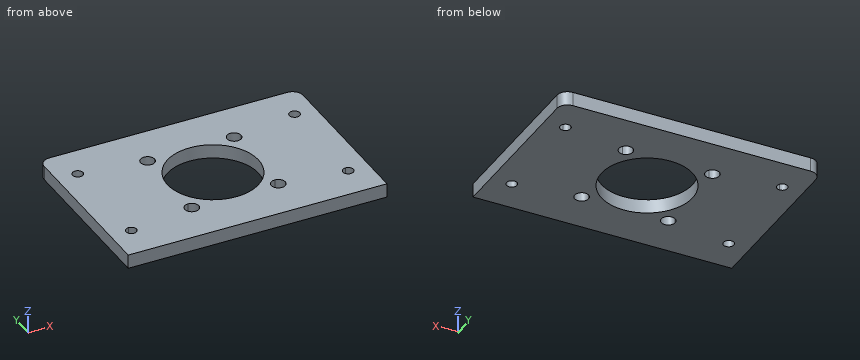
```python
from build123d import *

# Parameters (mm, degrees)
SKETCH_1_W            = 74
SKETCH_1_H            = 50
EXTRUDE_1_DEPTH       = 4
SKETCH_2_R            = 13
CUT_EXTRUDE_1_DEPTH   = 45.833023543
CUT_EXTRUDE_2_DEPTH   = 45.833023543
MIRROR_2_COPY_1_DEPTH = 45.833023543
CUT_EXTRUDE_3_DEPTH   = 45.833023543
MIRROR_4_COPY_1_DEPTH = 45.833023543
FILLET_2_R            = 3


with BuildPart() as part:
    # 草图1 → 凸台-拉伸1 (new body)
    with BuildSketch(Plane.XY):
        Rectangle(SKETCH_1_W, SKETCH_1_H)
    extrude(amount=EXTRUDE_1_DEPTH)

    # 草图2 → 切除-拉伸1 (cut, through all)
    with BuildSketch(Plane.XY.offset(4)):
        Circle(SKETCH_2_R)
    extrude(amount=-CUT_EXTRUDE_1_DEPTH, mode=Mode.SUBTRACT)

    # 草图3 → 切除-拉伸2 (cut, through all)
    with BuildSketch(Plane.XY.offset(4)):
        with BuildLine():
            ThreePointArc((10.374368671, 12.374368671), (10.960155108, 10.960155108), (12.374368671, 10.374368671))
            Line((12.374368671, 10.374368671), (12.374368671, 12.374368671))
            Line((12.374368671, 12.374368671), (10.374368671, 12.374368671))
        make_face()
        with BuildLine():
            Line((12.374368671, 12.374368671), (12.374368671, 10.374368671))
            ThreePointArc((12.374368671, 10.374368671), (13.788582233, 10.960155108), (14.374368671, 12.374368671))
            ThreePointArc((14.374368671, 12.374368671), (12.374368671, 14.374368671), (10.374368671, 12.374368671))
            Line((10.374368671, 12.374368671), (12.374368671, 12.374368671))
        make_face()
    cut_extrude_2 = extrude(amount=-CUT_EXTRUDE_2_DEPTH, mode=Mode.SUBTRACT)

    # 镜向1: 切除-拉伸2 across plane
    add(cut_extrude_2.mirror(Plane(origin=(0, 0, 0), x_dir=(0, 0, 1), z_dir=(1, 0, 0))), mode=Mode.SUBTRACT)

    # 镜向2: 切除-拉伸2 across plane
    add(cut_extrude_2.mirror(Plane.ZX), mode=Mode.SUBTRACT)

    # 镜向2 copy 1 sketch → 镜向2 copy 1 (cut, through all)
    with BuildSketch(Plane(origin=(0, 0, 4), x_dir=(-1, 0, 0), z_dir=(0, 0, 1))):
        with BuildLine():
            ThreePointArc((10.374368671, 12.374368671), (10.960155108, 10.960155108), (12.374368671, 10.374368671))
            Line((12.374368671, 10.374368671), (12.374368671, 12.374368671))
            Line((12.374368671, 12.374368671), (10.374368671, 12.374368671))
        make_face()
        with BuildLine():
            Line((12.374368671, 12.374368671), (12.374368671, 10.374368671))
            ThreePointArc((12.374368671, 10.374368671), (13.788582233, 10.960155108), (14.374368671, 12.374368671))
            ThreePointArc((14.374368671, 12.374368671), (12.374368671, 14.374368671), (10.374368671, 12.374368671))
            Line((10.374368671, 12.374368671), (12.374368671, 12.374368671))
        make_face()
    extrude(amount=-MIRROR_2_COPY_1_DEPTH, mode=Mode.SUBTRACT)

    # 草图4 → 切除-拉伸3 (cut, through all)
    with BuildSketch(Plane.XY.offset(4)):
        with BuildLine():
            ThreePointArc((-29.5, 15), (-32.060660172, 16.060660172), (-31, 13.5))
            Line((-31, 13.5), (-31, 15))
            Line((-31, 15), (-29.5, 15))
        make_face()
        with BuildLine():
            Line((-31, 15), (-31, 13.5))
            ThreePointArc((-31, 13.5), (-29.939339828, 13.939339828), (-29.5, 15))
            Line((-29.5, 15), (-31, 15))
        make_face()
    cut_extrude_3 = extrude(amount=-CUT_EXTRUDE_3_DEPTH, mode=Mode.SUBTRACT)

    # 镜向3: 切除-拉伸3 across plane
    add(cut_extrude_3.mirror(Plane(origin=(0, 0, 0), x_dir=(0, 0, 1), z_dir=(1, 0, 0))), mode=Mode.SUBTRACT)

    # 镜向4: 切除-拉伸3 across plane
    add(cut_extrude_3.mirror(Plane.ZX), mode=Mode.SUBTRACT)

    # 镜向4 copy 1 sketch → 镜向4 copy 1 (cut, through all)
    with BuildSketch(Plane(origin=(0, 0, 4), x_dir=(-1, 0, 0), z_dir=(0, 0, 1))):
        with BuildLine():
            ThreePointArc((-29.5, 15), (-32.060660172, 16.060660172), (-31, 13.5))
            Line((-31, 13.5), (-31, 15))
            Line((-31, 15), (-29.5, 15))
        make_face()
        with BuildLine():
            Line((-31, 15), (-31, 13.5))
            ThreePointArc((-31, 13.5), (-29.939339828, 13.939339828), (-29.5, 15))
            Line((-29.5, 15), (-31, 15))
        make_face()
    extrude(amount=-MIRROR_4_COPY_1_DEPTH, mode=Mode.SUBTRACT)

    # 圆角2
    fillet_2_edges = [part.edges().sort_by_distance(p)[0] for p in [
        (-37, 25, 2),
        (37, 25, 2),
    ]]
    fillet(fillet_2_edges, radius=FILLET_2_R)


solid = part.part
```
For this review, take the finished solid that the model builds, in its own axes (mm). Round coordinates to 2 decimals unless told otherwise and drop trailing zeros. Write each loop counter-clockwise with the first axis right and the second up, starting at its lowest first coordinate (ties: lowest second). Pieces come first, ordered by that corner, then holes. Notation, with made-up numbers: (-14.75, -39) -> (20.25, -39) arc R10 ccw to (20.25, -26) -> close; hole circle Ø8 at (-15.5, 35). An arc over 180 degrees is marked (long way). One line per question, with ' | ' between items. Start each with the question number.
(1) Add section A-A, the plane z = 0.75. Give the number of separate pieces and of enclosed holes in the cut face, plus the area to 3 significant figures.
(2) Insertion check: P1, Ø6, axis at x = 3, y = 11.5, coming from the -Z side. The pin has a flat end and moves straight along its axis. Give the tip position at first contact, or say it passes through.
(3) Add section B-B, the plane x = 0. Write out the cut boundary in (y, z), plus the area to 3 significant figures.
(4) For line 1 along X through (y, z) = (-15, 1.25); line 2 along Y through (x, z) = (-31, 1.2); line 3 along Y through (x, z) = (11, 3.3), list the stretches that pass through material, from the lowest coordinate up. Write a range as from..to.
(5) Add section C-C, the plane y = -6. Write out the cut boundary in (x, z).
(6) Add section D-D, the plane x = -11.5. Write out the cut boundary in (y, z).
Answer list:
1) separate pieces: 1 | enclosed holes: 9 | area: 3,090 mm²
2) P1: z = 0
3) outline: (-25, 0) -> (-13, 0) -> (-13, 4) -> (-25, 4) -> close; (13, 0) -> (25, 0) -> (25, 4) -> (13, 4) -> close | area: 96.0 mm²
4) line 1: -37..-32.5, -29.5..29.5, 32.5..37 | line 2: -25..-16.5, -13.5..13.5, 16.5..25 | line 3: -25..-13.83, -10.92..-6.93, 6.93..10.92, 13.83..25
5) outline: (-37, 0) -> (-11.53, 0) -> (-11.53, 4) -> (-37, 4) -> close; (11.53, 0) -> (37, 0) -> (37, 4) -> (11.53, 4) -> close
6) outline: (-25, 0) -> (-14.17, 0) -> (-14.17, 4) -> (-25, 4) -> close; (-10.58, 0) -> (-6.06, 0) -> (-6.06, 4) -> (-10.58, 4) -> close; (6.06, 0) -> (10.58, 0) -> (10.58, 4) -> (6.06, 4) -> close; (14.17, 0) -> (25, 0) -> (25, 4) -> (14.17, 4) -> close
